The listing builds one solid part. Answer for the finished solid, in the listing's coordinates (mm). A direction names the side the tool comes from. Coordinates: 2 decimals unless noted, no trailing zeros. Order: outer loops, then holes, each group sorted by start corner. A loop starts at its lowest first (then second) coordinate and runs counter-clockwise, first axis right, second up. Notation, with made-up numbers: (8.5, 46.25) -> (20.5, 46.25) arc R34 cw to (20.5, 81.25) -> close; hole circle Ø8 at (-29, -2.5). An arc over 180 degrees is marked (long way). Return JSON: item names as keys, results as strings.
from build123d import *

# Parameters (mm, degrees)
SKETCH_1_W                       = 218
SKETCH_1_H                       = 40
EXTRUDE_1_DEPTH                  = 2
SM_EDGE_FLANGE_1_STRIP_W         = 12
SM_EDGE_FLANGE_1_STRIP_H         = 2
SM_EDGE_FLANGE_1_STRIP_CUT_DEPTH = 40
SM_EDGE_FLANGE_1_DEPTH           = 40
SM_EDGE_FLANGE_2_STRIP_W         = 12
SM_EDGE_FLANGE_2_STRIP_H         = 2
SM_EDGE_FLANGE_2_STRIP_CUT_DEPTH = 40
SM_EDGE_FLANGE_2_DEPTH           = 40


# Sheet-metal steps are written as plain solids
with BuildPart() as part:
    # Sketch 1 → Бобышка-Вытянуть1 (new body)
    with BuildSketch(Plane(origin=(0, 0, 0), x_dir=(1, 0, 0), z_dir=(0, 1, 0))):
        with Locations((109, 20)):
            Rectangle(SKETCH_1_W, SKETCH_1_H)
    extrude(amount=EXTRUDE_1_DEPTH)

    # Ребро-кромка1 strip (across the edge) → Ребро-кромка1 strip cut (cut)
    with BuildSketch(Plane(origin=(0, 2, -40), x_dir=(1, 0, 0), z_dir=(0, 0, 1))):
        with Locations((-2, -1)):
            Rectangle(SM_EDGE_FLANGE_1_STRIP_W, SM_EDGE_FLANGE_1_STRIP_H)
    extrude(amount=SM_EDGE_FLANGE_1_STRIP_CUT_DEPTH, mode=Mode.SUBTRACT)

    # Ребро-кромка1 section (across the edge) → Ребро-кромка1 (add)
    with BuildSketch(Plane(origin=(0, 2, -40), x_dir=(1, 0, 0), z_dir=(0, 0, 1))):
        with BuildLine():
            Line((0, 2), (0, 38))
            Line((0, 38), (2, 38))
            Line((2, 38), (2, 2))
            ThreePointArc((2, 2), (2.585786438, 0.585786438), (4, 0))
            Line((4, 0), (4, -2))
            ThreePointArc((4, -2), (1.171572875, -0.828427125), (0, 2))
        make_face()
    extrude(amount=SM_EDGE_FLANGE_1_DEPTH)

    # Ребро-кромка2 strip (across the edge) → Ребро-кромка2 strip cut (cut)
    with BuildSketch(Plane(origin=(218, 2, 0), x_dir=(-1, 0, 0), z_dir=(0, 0, -1))):
        with Locations((-2, -1)):
            Rectangle(SM_EDGE_FLANGE_2_STRIP_W, SM_EDGE_FLANGE_2_STRIP_H)
    extrude(amount=SM_EDGE_FLANGE_2_STRIP_CUT_DEPTH, mode=Mode.SUBTRACT)

    # Ребро-кромка2 section (across the edge) → Ребро-кромка2 (add)
    with BuildSketch(Plane(origin=(218, 2, 0), x_dir=(-1, 0, 0), z_dir=(0, 0, -1))):
        with BuildLine():
            Line((0, 2), (0, 38))
            Line((0, 38), (2, 38))
            Line((2, 38), (2, 2))
            ThreePointArc((2, 2), (2.585786438, 0.585786438), (4, 0))
            Line((4, 0), (4, -2))
            ThreePointArc((4, -2), (1.171572875, -0.828427125), (0, 2))
        make_face()
    extrude(amount=SM_EDGE_FLANGE_2_DEPTH)


solid = part.part
1. Determine the mould class of faces 1 (the face through (108, 1, -40)), 2 (the face through (216, 22, -20)), 3 (the face through (1.203, 1.141, -20.28)) for opening direction X: pulls with the +X half, pulls with the -X half, needs draft (parallel to the pull), parting line crosses it, or undercut.
Answer block:
{"face 1": "needs draft", "face 2": "undercut", "face 3": "pulls with the -X half"}
2. This flat-tipped pin is pushed along its axis until it touches: pin 1 Ø3 at (x, z) = (92, -19) entering from +Y. Where does it stop, or does it pass through?
Answer block:
{"pin 1": "stops at y = 2"}
3. The part is cut by section A-A on y = 26. Give the vertices of the cut face in (x, z).
Answer block:
{"outline": "(0, -40) -> (2, -40) -> (2, 0) -> (0, 0) -> close; (216, -40) -> (218, -40) -> (218, 0) -> (216, 0) -> close"}
4. The part is cut by section C-C on x = 174. Give the vertices of the cut face in (y, z).
Answer block:
{"outline": "(0, -40) -> (2, -40) -> (2, 0) -> (0, 0) -> close"}
5. For faces 4 (the face through (108, 2, -20)), 5 (the face through (108, 1, 0)), determine the directions among +Z, -Z, +X, -X, +Y, -Y from which every point of the face is accessible in a straight line to the end or side of a thin tool.
Answer block:
{"face 4": "+Z, -Z, +Y", "face 5": "+Z, +X, -X, +Y, -Y"}
6. Consider line 1 (X direction, y = 26.5, z = -15); line 2 (Y direction, x = 46, z = -23.5); line 3 (X direction, y = 3.5, z = -18.5). Determine where each line is inside the solid, lowest interval first. Write a range as from..to.
Answer block:
{"line 1": "x = 0..2, 216..218", "line 2": "y = 0..2", "line 3": "x = 0.03..2.06, 215.94..217.97"}
7. The part is cut by section B-B on z = -32.5. Give the vertices of the cut face in (x, y).
Answer block:
{"outline": "(0, 4) arc R4 ccw to (4, 0) -> (214, 0) arc R4 ccw to (218, 4) -> (218, 40) -> (216, 40) -> (216, 4) arc R2 cw to (214, 2) -> (4, 2) arc R2 cw to (2, 4) -> (2, 40) -> (0, 40) -> close"}
